Input: dimensioned drawing with shaded views. Units: mm. Origin: part minimum x, y, z. Give positions to 0.01 mm unless a question says otherwise; leave off trailing zeros. Write each loop counter-clockwise with the first axis right and the second up, starting at its lowest first coordinate (ties: lowest second). Pieces come first, ordered by that corner, then holes. Notation, with made-up numbers: (35, 83) - (46, 83) arc R19 ccw to (46, 96) - close; hole circle Ø7 at (17, -13.5). An arc over 180 degrees is marked (long way). Answer as a JSON object with one key per item and string values. Group by question number.
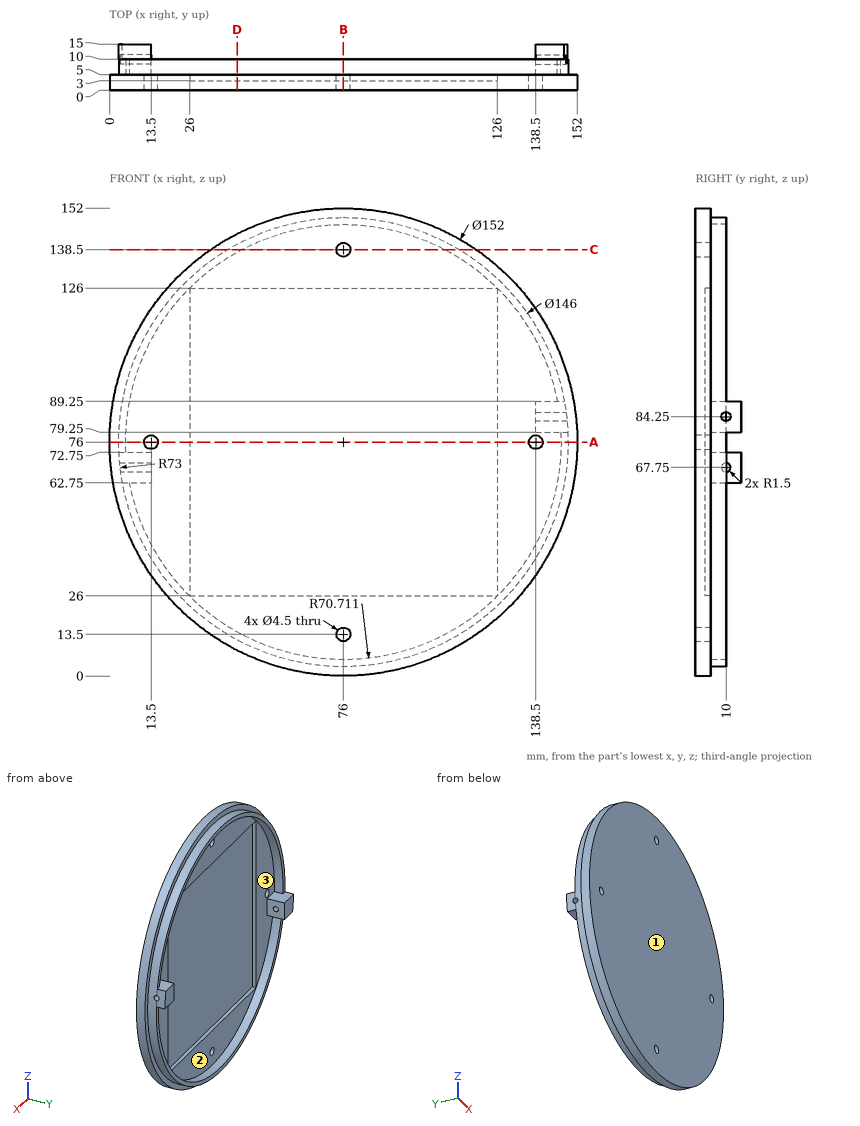
Q1. Section A-A on z = 76. Return the cut outline in (x, y).
Q2. Ray query, probe 1 along X at (y, z) = (2.05, 76); probe 2 along X at (y, z) = (3.8, 76); probe 3 along Z at (x, y) = (76, 8.5). Return the intervals inside material, ascending. Write a range as [from, to].
Q3. Draft query along X for the marked faces 1, 2 and 3. Return one class per face: released by +X, released by -X, zero draft, split by the parting line, or undercut.
Q4. Section D-D on x = 41.5. Return the cut outline in (y, z), then the cut area to 3 significant figures.
Q5. Section B-B on x = 76. Return the cut outline in (y, z), then the cut area to 3 significant figures.
Q6. Section C-C on z = 138.5. Return the cut outline in (x, y).
Q7. First-contact query: pin 1 Ø3 at (y, z) = (9, 85.5) entering from -X; pin 2 Ø4.5 at (x, y) = (143, 9) entering from +Z; pin 3 Ø6 at (x, y) = (114, 12.5) entering from -Z; pin 4 Ø5 at (x, y) = (54, 13) entering from -Z. Flat tips, straight axial feed; report the tip coordinate or a pass-through.
Taken from the geometry:
{
 "1": {"outline": "(0, 0) - (11.25, 0) - (11.25, 5) - (5.29, 5) - (5.29, 10) - (3, 10) - (3, 5) - (0, 5) - close; (15.75, 0) - (136.25, 0) - (136.25, 5) - (126, 5) - (126, 3) - (26, 3) - (26, 5) - (15.75, 5) - close; (140.75, 0) - (152, 0) - (152, 5) - (149, 5) - (149, 10) - (146.71, 10) - (146.71, 5) - (140.75, 5) - close"},
 "2": {"probe 1": "x = [0, 11.25], [15.75, 136.25], [140.75, 152]", "probe 2": "x = [0, 11.25], [15.75, 26], [126, 136.25], [140.75, 152]", "probe 3": "z = [3, 5.29], [146.71, 149]"},
 "3": {"face 1": "zero draft", "face 2": "undercut", "face 3": "undercut"},
 "4": {"outline": "(0, 8.28) - (5, 8.28) - (5, 11.67) - (10, 11.67) - (10, 14.28) - (5, 14.28) - (5, 26) - (3, 26) - (3, 126) - (5, 126) - (5, 137.72) - (10, 137.72) - (10, 140.33) - (5, 140.33) - (5, 143.72) - (0, 143.72) - close", "area": "503 mm²"},
 "5": {"outline": "(0, 0) - (5, 0) - (5, 3) - (10, 3) - (10, 5.29) - (5, 5.29) - (5, 11.25) - (0, 11.25) - close; (0, 15.75) - (5, 15.75) - (5, 26) - (3, 26) - (3, 126) - (5, 126) - (5, 136.25) - (0, 136.25) - close; (0, 140.75) - (5, 140.75) - (5, 146.71) - (10, 146.71) - (10, 149) - (5, 149) - (5, 152) - (0, 152) - close", "area": "538 mm²"},
 "6": {"outline": "(32.76, 0) - (73.75, 0) - (73.75, 5) - (42.93, 5) - (42.93, 10) - (38.28, 10) - (38.28, 5) - (32.76, 5) - close; (78.25, 0) - (119.24, 0) - (119.24, 5) - (113.72, 5) - (113.72, 10) - (109.07, 10) - (109.07, 5) - (78.25, 5) - close"},
 "7": {"pin 1": "stops at x = 3.44", "pin 2": "stops at z = 109.71", "pin 3": "stops at z = 12.69", "pin 4": "passes through"}
}
